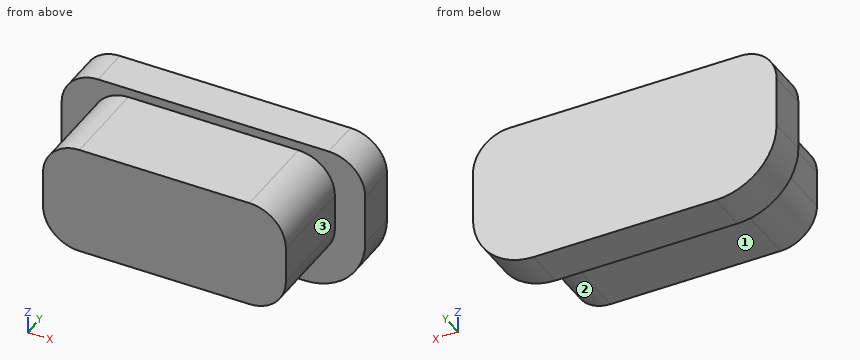
from build123d import *

# Parameters (mm, degrees)
EXTRUDE031_DEPTH = 1
EXTRUDE030_DEPTH = 2.75


with BuildPart() as extrude031:
    # Sketch034 → Extrude031 (new body)
    with BuildSketch(Plane.XZ):
        with BuildLine():
            ThreePointArc((11.7, 16.35), (11.063604, 16.086396), (10.8, 15.45))
            Line((10.8, 14.2), (10.8, 15.45))
            ThreePointArc((10.8, 14.2), (11.23934, 13.13934), (12.3, 12.7))
            Line((16.8, 12.7), (12.3, 12.7))
            ThreePointArc((16.8, 12.7), (17.86066, 13.13934), (18.3, 14.2))
            Line((18.3, 15.45), (18.3, 14.2))
            ThreePointArc((18.3, 15.45), (18.036396, 16.086396), (17.4, 16.35))
            Line((11.7, 16.35), (17.4, 16.35))
        make_face()
    extrude(amount=EXTRUDE031_DEPTH)


with BuildPart() as extrude031_1:
    # Extrude031 placement: moved
    add(extrude031.part.moved(Location((0, 2.5, 0))))


with BuildPart() as button002:
    # Sketch033 → Extrude030 (new body)
    with BuildSketch(Plane.XZ):
        with BuildLine():
            ThreePointArc((12.75, 16.23), (12.113604, 15.966396), (11.85, 15.33))
            Line((11.85, 14.43), (11.85, 15.33))
            ThreePointArc((11.85, 14.43), (12.113604, 13.793604), (12.75, 13.53))
            Line((16.95, 13.53), (12.75, 13.53))
            ThreePointArc((16.95, 13.53), (17.586396, 13.793604), (17.85, 14.43))
            Line((17.85, 15.33), (17.85, 14.43))
            ThreePointArc((17.85, 15.33), (17.586396, 15.966396), (16.95, 16.23))
            Line((12.75, 16.23), (16.95, 16.23))
        make_face()
    extrude(amount=EXTRUDE030_DEPTH)


with BuildPart() as button002_1:
    # Extrude030 placement: moved
    add(button002.part.moved(Location((-0.3, 2, -0.1))))

    # Fusion033: union Extrude031
    add(extrude031_1.part)


with BuildPart() as button002_2:
    # Fusion033 placement: moved
    add(button002_1.part.moved(Location((32.45, 0, 0))))


solid = button002_2.part
Can you work these out from the model? Positions are in its coordinate system, mm. Face numbers are marked on the shaded views. A direction names the side the tool comes from. Give positions to 0.01 mm unless a question says otherwise; leave off trailing zeros. Loops run counter-clockwise (first coordinate to the right, second up) from the corner with the lowest first, then second, coordinate; pieces in that order, holes last. Notation, with made-up numbers: (88.5, -5.5) - (95.5, -5.5) arc R21 ccw to (95.5, 2.5) - close; hole circle Ø3 at (-5.5, 7). An arc over 180 degrees is marked (long way). Return JSON: item names as keys, results as strings.
1. For the marked faces 1, 2 and 3, which set-ups out of +Z, -Z, +X, -X, +Y, -Y let a thin tool reach every point of the face, with its end or its side?
Output values:
{"face 1": "-Z, +X, -X, -Y", "face 2": "-Z, +X, -Y", "face 3": "+Z, -Z, +X, -Y"}
2. I want a section at B-B on x = 47.5. Please give me the cut outline in (y, z), and give its area (4 significant figures).
Output values:
{"outline": "(-0.75, 13.43) - (1.5, 13.43) - (1.5, 12.7) - (2.5, 12.7) - (2.5, 16.35) - (1.5, 16.35) - (1.5, 16.13) - (-0.75, 16.13) - close", "area": "9.725 mm²"}
3. I want a section at C-C on z = 13.3. Please give me the cut outline in (x, y).
Output values:
{"outline": "(43.55, 1.5) - (50.45, 1.5) - (50.45, 2.5) - (43.55, 2.5) - close"}
4. I'm going to push flat-ended pins straight in: pin 1 Ø1.8 at (x, y) = (47, 0.5) entering from +Z; pin 2 Ø1.1 at (x, y) = (46, 0) entering from -Z; pin 3 Ø1.5 at (y, z) = (-0.5, 13) entering from +X. Where does each tip first touch, or does it pass through?
Output values:
{"pin 1": "stops at z = 16.13", "pin 2": "stops at z = 13.43", "pin 3": "stops at x = 49.79"}
5. If I drill on line 1 (X direction, y = 0.7, z = 14.4); line 2 (Z direction, x = 47.25, y = -0.6); line 3 (Y direction, x = 44.5, z = 13.4), over which ranges is the centre line in solid material (lowest first)?
Output values:
{"line 1": "x = 44 to 50", "line 2": "z = 13.43 to 16.13", "line 3": "y = 1.5 to 2.5"}
6. I want a section at A-A on y = 1.8. Please give me the cut outline in (x, z).
Output values:
{"outline": "(43.25, 14.2) arc R1.5 ccw to (44.75, 12.7) - (49.25, 12.7) arc R1.5 ccw to (50.75, 14.2) - (50.75, 15.45) arc R0.9 ccw to (49.85, 16.35) - (44.15, 16.35) arc R0.9 ccw to (43.25, 15.45) - close"}
